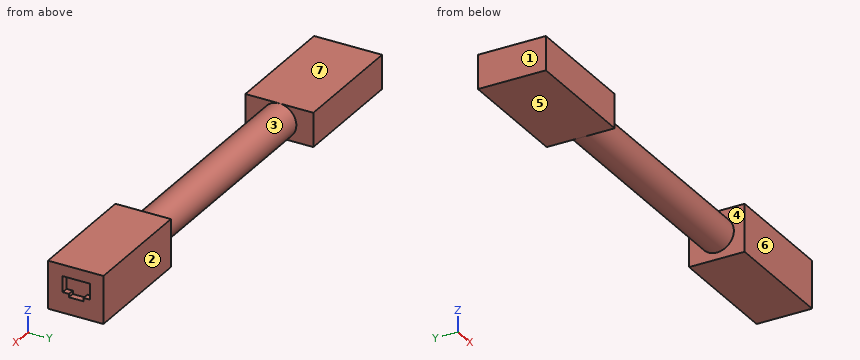
from build123d import *

# Parameters (mm, degrees)
F0_W     = 24.5
F0_H     = 21
F1_DEPTH = 52
F2_R     = 7.5
F3_DEPTH = 105
F4_W     = 30
F4_H     = 15
F5_DEPTH = 53
F6_DEPTH = 3


with BuildPart() as f1:
    # F0 (on Right) → F1 (new body)
    with BuildSketch(Plane.YZ):
        Rectangle(F0_W, F0_H)
        Polygon((-3, -1.5), (-5.75, -1.5), (-5.75, 5.5), (6.25, 5.5), (6.25, -1.5), (3.5, -1.5), (3.5, -3), (-3, -3), align=None, mode=Mode.SUBTRACT)
        Polygon((-5.75, 5.5), (-5.75, -1.5), (-3, -1.5), (-3, -3), (3.5, -3), (3.5, -1.5), (6.25, -1.5), (6.25, 5.5), align=None)
    extrude(amount=-F1_DEPTH)

    # F2 (on face) → F3 (join)
    with BuildSketch(Plane(origin=(-52, 0, 0), x_dir=(0, -1, 0), z_dir=(-1, 0, 0))):
        Circle(F2_R)
    extrude(amount=F3_DEPTH)

    # F4 (on face) → F5 (join)
    with BuildSketch(Plane(origin=(-157, 0, 0), x_dir=(0, -1, 0), z_dir=(-1, 0, 0))):
        Rectangle(F4_W, F4_H)
    extrude(amount=F5_DEPTH)

    # F0 (on Right) → F6 (cut)
    with BuildSketch(Plane.YZ):
        Polygon((-5.75, 5.5), (-5.75, -1.5), (-3, -1.5), (-3, -3), (3.5, -3), (3.5, -1.5), (6.25, -1.5), (6.25, 5.5), align=None)
    extrude(amount=-F6_DEPTH, mode=Mode.SUBTRACT)


solid = f1.part
Input: part model. Units: mm. Frame: model coordinates. Face numbers are marked on the shaded views. A direction names the side the tool comes from. Coordinates: 2 decimals unless noted, no trailing zeros. Loops run counter-clockwise (first coordinate to the right, second up) from the corner with the lowest first, then second, coordinate; pieces in that order, holes last. Notation, with made-up numbers: (82, 76.25) - (95, 76.25) arc R8 ccw to (95, 81.25) - close; hole circle Ø1 at (52.25, -38.75). An arc over 180 degrees is marked (long way). Answer in a Markdown table with one row per item. Add a question column.
Item 1: Section query C-C on x = -183. Return the cut outline in (y, z), then the cut area to 3 significant figures.
Item 2: Section query B-B on x = -136.5. Return the cut outline in (y, z), then the cut area to 3 significant figures.
Item 3: Mould query, pull axis X, two halves, no side actions, for the marked faces 1, 2 and 3. Classes: released by +X, released by -X, zero draft, split by the parting line, or undercut.
Item 4: Contact query for flat-ended pins moving along their axis: P1, Ø6, axis at x = -124, z = -4, coming from the +Y side; P2, Ø1.5, axis at x = -108.5, y = 4.5, coming from the -Z side; P3, Ø15, axis at x = -175, y = 6.5, coming from the -Z side. Output: stop coordinate, or through.
Item 5: Line query: line 1 along X through (y, z) = (-9.5, 4); line 2 along X through (y, z) = (6, -9); line 3 along Y through (x, z) = (-8.5, 8). Output: solid intervals per line, ascending. Write a range as [from, to].
Item 6: Section query A-A on z = 2. Return the cut outline in (x, y), then the cut area to 3 significant figures.
Item 7: Access query for the marked faces 4, 5, 6 and 7. Directions: +Z, -Z, +X, -X, +Y, -Y. A direction counts if a zero-diameter tool reaches every point of the face in a straight line with its end or side. Return the directions, or none.
Recorded:
| question | item | result |
|---|---|---|
| 1 | outline | (-15, -7.5) - (15, -7.5) - (15, 7.5) - (-15, 7.5) - close |
| 1 | area | 450 mm^2 |
| 2 | outline | circle Ø15 at (0, 0) |
| 2 | area | 177 mm^2 |
| 3 | face 1 | released by -X |
| 3 | face 2 | zero draft |
| 3 | face 3 | undercut |
| 4 | P1 | y = 7.43 |
| 4 | P2 | z = -6.5 |
| 4 | P3 | z = -7.5 |
| 5 | line 1 | [-210, -157], [-52, 0] |
| 5 | line 2 | [-52, 0] |
| 5 | line 3 | [-12.25, 12.25] |
| 6 | outline | (-210, -15) - (-157, -15) - (-157, -7.23) - (-52, -7.23) - (-52, -12.25) - (0, -12.25) - (0, -5.75) - (-3, -5.75) - (-3, 6.25) - (0, 6.25) - (0, 12.25) - (-52, 12.25) - (-52, 7.23) - (-157, 7.23) - (-157, 15) - (-210, 15) - close |
| 6 | area | 4,350 mm^2 |
| 7 | face 4 | none |
| 7 | face 5 | -Z, -X, +Y, -Y |
| 7 | face 6 | +Z, -Z, +X, -Y |
| 7 | face 7 | +Z, -X, +Y, -Y |
